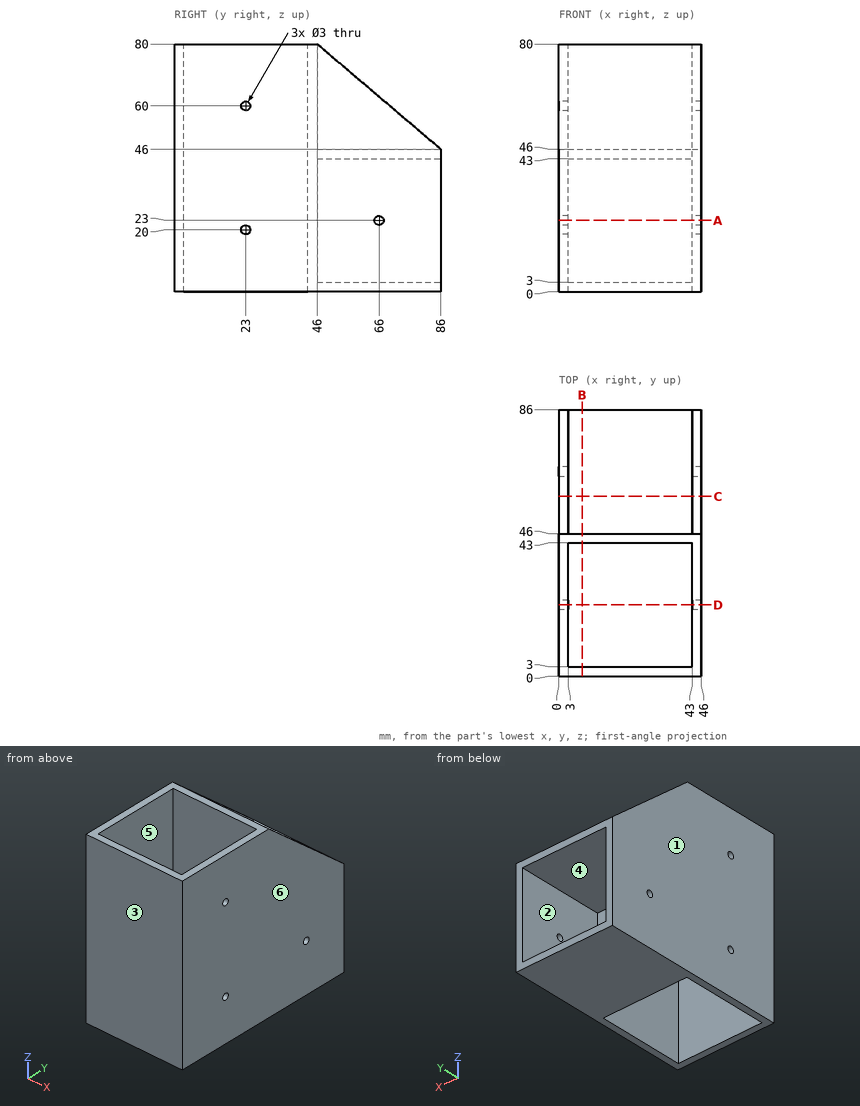
For this review, use the dimensioned drawing (mm, ordinates from the lowest corner) and the shaded views. A direction names the side the tool comes from. Round coordinates to 2 decimals unless told otherwise and drop trailing zeros. Order: outer loops, then holes, each group sorted by start corner. A loop starts at its lowest first (then second) coordinate and runs counter-clockwise, first axis right, second up. Notation, with made-up numbers: (40.5, -15) -> (96.5, -15) arc R25 ccw to (96.5, 11) -> close; hole circle Ø10 at (-18, 57.25). An arc over 180 degrees is marked (long way). One line per item, written item: value. Start each with the question number.
Q1. Clearance check with flat-ended pins moving along their axes: pin 1 Ø1.8 at (y, z) = (66, 23) entering from -X; pin 2 Ø6 at (x, z) = (23.5, 49.5) entering from +Y; pin 3 Ø10 at (x, y) = (41.5, 75) entering from +Z. State where each tip first meets the part, or that it passes through.
Q2. Mouldability with a two-part tool opening along X and no side actions: class the marked faces 1, 2 and 3 as released by +X, released by -X, zero draft, split by the parting line, or undercut.
Q3. Take a section at C-C (y = 58). Write out the cut boundary in (x, z).
Q4. Wall thickness on line 1 (Z direction, x = 43.8, y = 23); line 2 (X direction, y = 6.5, z = 29): over which ranges is each line inside the solid? List them lowest first.
Q5. Take a section at A-A (z = 23). Write out the cut boundary in (x, y).
Q6. Take a section at B-B (x = 7.5). Write out the cut boundary in (y, z).
Q7. Take a section at D-D (y = 23). Write out the cut boundary in (x, z), and give its area (3 significant figures).
Q8. Machinability: for the marked faces 4, 5 and 6, which of the approach directions +Z, -Z, +X, -X, +Y, -Y give a long, thin tool a straight path to every point of the face, cutting with its end or side? Answer none if there is none.
Reported:
1. pin 1: passes through
1. pin 2: stops at y = 46
1. pin 3: stops at z = 59.4
2. face 1: released by -X
2. face 2: undercut
2. face 3: zero draft
3. outline: (0, 0) -> (46, 0) -> (46, 69.8) -> (43, 69.8) -> (43, 46) -> (3, 46) -> (3, 69.8) -> (0, 69.8) -> close; hole (3, 3) -> (43, 3) -> (43, 43) -> (3, 43) -> close
4. line 1: z = 0 to 18.5, 21.5 to 58.5, 61.5 to 80
4. line 2: x = 0 to 3, 43 to 46
5. outline: (0, 0) -> (46, 0) -> (46, 64.5) -> (43, 64.5) -> (43, 46) -> (3, 46) -> (3, 64.5) -> (0, 64.5) -> close; (0, 67.5) -> (3, 67.5) -> (3, 86) -> (0, 86) -> close; (43, 67.5) -> (46, 67.5) -> (46, 86) -> (43, 86) -> close; hole (3, 3) -> (43, 3) -> (43, 43) -> (3, 43) -> close
6. outline: (0, 0) -> (3, 0) -> (3, 80) -> (0, 80) -> close; (43, 0) -> (86, 0) -> (86, 3) -> (46, 3) -> (46, 43) -> (86, 43) -> (86, 46) -> (46, 46) -> (46, 80) -> (43, 80) -> close
7. outline: (0, 0) -> (3, 0) -> (3, 18.5) -> (0, 18.5) -> close; (0, 21.5) -> (3, 21.5) -> (3, 58.5) -> (0, 58.5) -> close; (0, 61.5) -> (3, 61.5) -> (3, 80) -> (0, 80) -> close; (43, 0) -> (46, 0) -> (46, 18.5) -> (43, 18.5) -> close; (43, 21.5) -> (46, 21.5) -> (46, 58.5) -> (43, 58.5) -> close; (43, 61.5) -> (46, 61.5) -> (46, 80) -> (43, 80) -> close
7. area: 444 mm2
8. face 4: +Y
8. face 5: +Z, -Z
8. face 6: +Z, -Z, +X, +Y, -Y
